Can you work these out from the drawing? Everything is in mm from the part's minimum corner. Coordinates: 2 decimals unless noted, no trailing zeros. Loops run counter-clockwise (first coordinate to the right, second up) from the corner with the lowest first, then second, coordinate; pieces in that order, holes last. Notation, with made-up numbers: (26.25, -32.75) -> (31.25, -32.75) arc R34 cw to (31.25, 3.25) -> close; hole circle Ø10 at (-19.5, 89). An arc over 180 degrees is marked (long way). Put each result on its own line as item: value. Start each with the question number.
Item 1: If we section it at A-A on x = 3: Please give me the cut outline in (y, z).
Item 2: If we section it at C-C on x = 33: Please give me the cut outline in (y, z).
Item 3: Please list where these lines run through material, in increasing order: L1, parallel to X at y = 3, z = 1.5 (1 decimal); L2, parallel to X at y = 2, z = 0.4; L3, parallel to Y at x = 18, z = 0.3. Write a range as from..to.
Item 4: If we section it at B-B on z = 1.6: Please give me the cut outline in (x, y) (1 decimal), plus the area to 3 significant figures.
Item 5: If we section it at D-D on x = 22: Please give me the cut outline in (y, z).
Item 6: Will these pins go through, and if not, where does the flat tip stop? P1, Ø1, axis at x = 21.5, z = 1.5, coming from the -Y side; P2, Ø1, axis at x = 9.5, y = 6.5, coming from the -Z side; P3, Ø0.6, axis at x = 23.5, z = 1, coming from the +Y side.
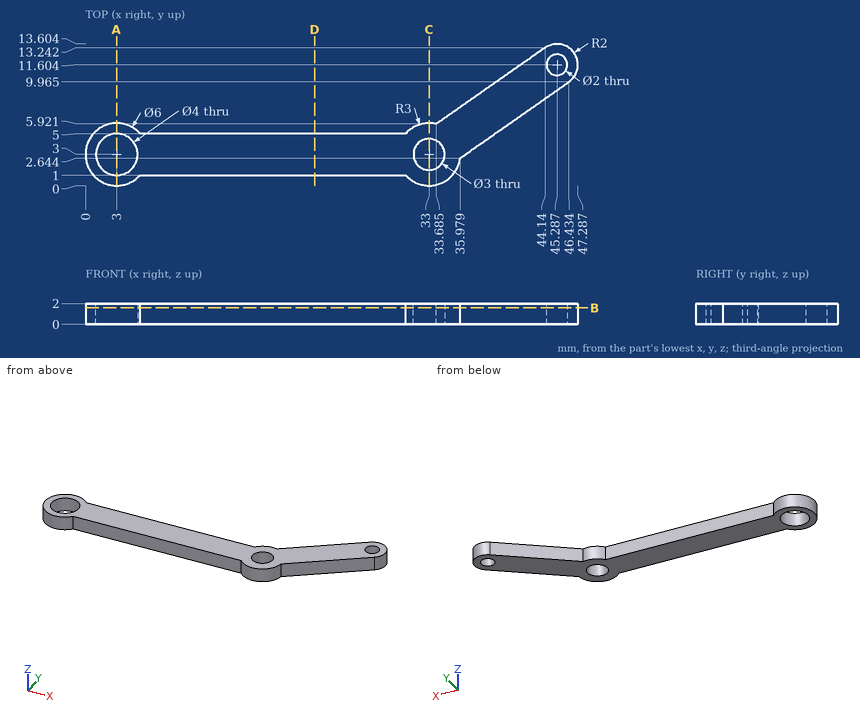
Solutions:
1. outline: (0, 0) -> (1, 0) -> (1, 2) -> (0, 2) -> close; (5, 0) -> (6, 0) -> (6, 2) -> (5, 2) -> close
2. outline: (0, 0) -> (1.5, 0) -> (1.5, 2) -> (0, 2) -> close; (4.5, 0) -> (6, 0) -> (6, 2) -> (4.5, 2) -> close
3. L1: 0..1, 5..31.5, 34.5..36.5
3. L2: 0.17..1.27, 4.73..31.88, 34.12..35.83
3. L3: 1..5
4. outline: (5.2, 1) -> (30.8, 1) arc R3 ccw to (36, 2.6) -> (46.4, 10) arc R2 ccw to (44.1, 13.2) -> (33.7, 5.9) arc R3 ccw to (30.8, 5) -> (5.2, 5) arc R3 ccw (long way) to start; hole circle Ø4 at (3, 3); hole circle Ø3 at (33, 3); hole circle Ø2 at (45.3, 11.6)
4. area: 187 mm^2
5. outline: (1, 0) -> (5, 0) -> (5, 2) -> (1, 2) -> close
6. P1: y = 1
6. P2: through
6. P3: y = 5
